from build123d import *

# Parameters (mm, degrees)
SKETCH_1_W                = 28
SKETCH_1_H                = 20
SKETCH_2_W                = 40
SKETCH_2_H                = 20
SKETCH_3_W                = 40
SKETCH_3_H                = 20
EXTRUDE_1_DEPTH           = 24
SKETCH_4_W                = 19
SKETCH_4_H                = 20
CUT_EXTRUDE_1_DEPTH       = 30
HOLE_WIZARD_M31_D         = 2.5
HOLE_WIZARD_M31_DEPTH     = 9
HOLE_WIZARD_M31_TIP       = 0.751075774
SKETCH_11_R               = 7
CUT_EXTRUDE_3_DEPTH       = 32
SKETCH_12_R               = 2
CUT_EXTRUDE_4_DEPTH       = 30
SKETCH_13_R               = 1.25
CUT_EXTRUDE_5_DEPTH       = 22
CUT_EXTRUDE_6_REACH       = 42
SKETCH_14_R               = 1.6
SKETCH_15_R               = 4
CUT_EXTRUDE_7_DEPTH       = 21
CHAMFER_1_SIZE            = 0.5
HOLE_WIZARD_M41_D         = 3.3
HOLE_WIZARD_M41_DEPTH     = 10
HOLE_WIZARD_M41_TIP       = 0.991420021
SKETCH_21_R               = 2.5
CUT_EXTRUDE_8_DEPTH       = 20
CUT_EXTRUDE_9_REACH       = 64
SKETCH_22_R               = 1.25
SKETCH_23_W               = 12.954085538
SKETCH_23_H               = 2
CUT_EXTRUDE_10_DEPTH      = 2
CUT_EXTRUDE_10_DEPTH_BACK = 2


with BuildPart() as part:
    # Эскиз1 → По сечениям1 section 0
    with BuildSketch(Plane(origin=(0, 0, 0), x_dir=(1, 0, 0), z_dir=(0, 1, 0))):
        with Locations((14, 10)):
            Rectangle(SKETCH_1_W, SKETCH_1_H)
    # Эскиз2 → По сечениям1 section 1
    with BuildSketch(Plane(origin=(0, -38, 0), x_dir=(1, 0, 0), z_dir=(0, 1, 0))):
        with Locations((20, 10)):
            Rectangle(SKETCH_2_W, SKETCH_2_H)
    loft()

    # Эскиз3 → Бобышка-Вытянуть1 (add)
    with BuildSketch(Plane.XZ.offset(38)):
        with Locations((20, -10)):
            Rectangle(SKETCH_3_W, SKETCH_3_H)
    extrude(amount=EXTRUDE_1_DEPTH)

    # Эскиз4 → Вырез-Вытянуть1 (cut)
    with BuildSketch(Plane.XZ.offset(62)):
        with Locations((9.5, -10)):
            Rectangle(SKETCH_4_W, SKETCH_4_H)
    extrude(amount=-CUT_EXTRUDE_1_DEPTH, mode=Mode.SUBTRACT)

    # Отверстие обработанное метчиком M31
    with Locations(Plane(origin=(0, 0, 0), x_dir=(1, 0, 0), z_dir=(0, 1, 0))):
        with Locations((3, 3), (3, 17), (24, 17), (24, 3)):
            Hole(HOLE_WIZARD_M31_D / 2, depth=HOLE_WIZARD_M31_DEPTH)
            with Locations((0, 0, -(HOLE_WIZARD_M31_DEPTH + HOLE_WIZARD_M31_TIP / 2))):  # 118° drill point
                Cone(0, HOLE_WIZARD_M31_D / 2, HOLE_WIZARD_M31_TIP, mode=Mode.SUBTRACT)

    # Эскиз11 → Вырез-Вытянуть3 (cut)
    with BuildSketch(Plane(origin=(0, 0, 0), x_dir=(1, 0, 0), z_dir=(0, 1, 0))):
        with Locations((10, 10)):
            Circle(SKETCH_11_R)
    extrude(amount=-CUT_EXTRUDE_3_DEPTH, mode=Mode.SUBTRACT)

    # Эскиз12 → Вырез-Вытянуть4 (cut)
    with BuildSketch(Plane(origin=(0, 0, 0), x_dir=(1, 0, 0), z_dir=(0, 1, 0))):
        with Locations((24, 10)):
            Circle(SKETCH_12_R)
    extrude(amount=-CUT_EXTRUDE_4_DEPTH, mode=Mode.SUBTRACT)

    # Эскиз13 → Вырез-Вытянуть5 (cut)
    with BuildSketch(Plane(origin=(0, -30, 0), x_dir=(1, 0, 0), z_dir=(0, 1, 0))):
        with Locations((24, 10)):
            Circle(SKETCH_13_R)
    extrude(amount=-CUT_EXTRUDE_5_DEPTH, mode=Mode.SUBTRACT)

    # Эскиз14 → Вырез-Вытянуть6 (cut, up to next)
    with BuildSketch(Plane.ZY, mode=Mode.PRIVATE) as cut_extrude_6_sk1:
        with Locations((-13, -17)):
            Circle(SKETCH_14_R)
    cut_extrude_6_tool1 = extrude(cut_extrude_6_sk1.sketch, amount=-CUT_EXTRUDE_6_REACH, mode=Mode.PRIVATE) & part.part
    add(cut_extrude_6_tool1.solids().sort_by_distance((0, -17, -13))[0], mode=Mode.SUBTRACT)
    # Эскиз14 → Вырез-Вытянуть6 (cut, up to next)
    with BuildSketch(Plane.ZY, mode=Mode.PRIVATE) as cut_extrude_6_sk2:
        with Locations((-7, -17)):
            Circle(SKETCH_14_R)
    cut_extrude_6_tool2 = extrude(cut_extrude_6_sk2.sketch, amount=-CUT_EXTRUDE_6_REACH, mode=Mode.PRIVATE) & part.part
    add(cut_extrude_6_tool2.solids().sort_by_distance((0, -17, -7))[0], mode=Mode.SUBTRACT)

    # Эскиз15 → Вырез-Вытянуть7 (cut)
    with BuildSketch(Plane(origin=(40, 0, 0), x_dir=(0, 0, -1), z_dir=(1, 0, 0))):
        with Locations((10, -52)):
            Circle(SKETCH_15_R)
    extrude(amount=-CUT_EXTRUDE_7_DEPTH, mode=Mode.SUBTRACT)

    # Фаска1
    chamfer_1_edges = [part.edges().sort_by_distance(p)[0] for p in [
        (40, -52, -6),
    ]]
    chamfer(chamfer_1_edges, length=CHAMFER_1_SIZE)

    # Отверстие обработанное метчиком M41
    with Locations(Plane(origin=(0, -62, 0), x_dir=(-1, 0, 0), z_dir=(0, -1, 0))):
        with Locations((-32, 10), (-24, 10)):
            Hole(HOLE_WIZARD_M41_D / 2, depth=HOLE_WIZARD_M41_DEPTH)
            with Locations((0, 0, -(HOLE_WIZARD_M41_DEPTH + HOLE_WIZARD_M41_TIP / 2))):  # 118° drill point
                Cone(0, HOLE_WIZARD_M41_D / 2, HOLE_WIZARD_M41_TIP, mode=Mode.SUBTRACT)

    # Эскиз21 → Вырез-Вытянуть8 (cut)
    with BuildSketch(Plane.XY):
        with Locations((32, -42)):
            Circle(SKETCH_21_R)
    extrude(amount=-CUT_EXTRUDE_8_DEPTH, mode=Mode.SUBTRACT)

    # Эскиз22 → Вырез-Вытянуть9 (cut, up to next)
    with BuildSketch(Plane.XZ.offset(62), mode=Mode.PRIVATE) as cut_extrude_9_sk1:
        with Locations((32, -10)):
            Circle(SKETCH_22_R)
    cut_extrude_9_tool1 = extrude(cut_extrude_9_sk1.sketch, amount=-CUT_EXTRUDE_9_REACH, mode=Mode.PRIVATE) & part.part
    add(cut_extrude_9_tool1.solids().sort_by_distance((32, -62, -10))[0], mode=Mode.SUBTRACT)

    # Эскиз23 → Вырез-Вытянуть10 (cut, two sides)
    with BuildSketch(Plane.XY.offset(-10)) as cut_extrude_10_sk:
        with Locations((17.522957231, -1)):
            Rectangle(SKETCH_23_W, SKETCH_23_H)
    extrude(amount=CUT_EXTRUDE_10_DEPTH, mode=Mode.SUBTRACT)
    extrude(cut_extrude_10_sk.sketch, amount=-CUT_EXTRUDE_10_DEPTH_BACK, mode=Mode.SUBTRACT)


solid = part.part
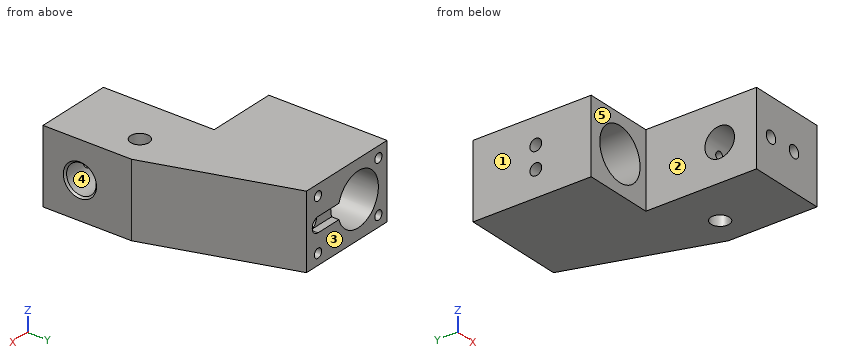
Can you work these out from the model? Positions are in its coordinate system, mm. Face numbers are marked on the shaded views. A direction names the side the tool comes from. Round coordinates to 2 decimals unless told otherwise and drop trailing zeros. Write each loop counter-clockwise with the first axis right and the second up, starting at its lowest first coordinate (ties: lowest second). Pieces come first, ordered by that corner, then holes. Notation, with made-up numbers: (-7.75, 67.5) - (-0.75, 67.5) arc R16 cw to (-0.75, 93.5) - close; hole circle Ø6 at (49.25, 16). An arc over 180 degrees is marked (long way). Write each question's results on one line, items separated by ' | '. Start each with the question number.
1) Suppose I cut it at A-A (y = -42). List the corners of the cut face in (x, z) for me.
2) Suppose I cut it at B-B (x = 10). List the corners of the cut face in (y, z) for me, and give its area (3 significant figures).
3) Please list where these lines run through material, in increasing order: line 1 (Y direction, x = 1.2, z = -13); line 2 (Z direction, x = 24, y = -7); line 3 (X direction, y = -45.35, z = -10).
4) Which directions (+Z, -Z, +X, -X, +Y, -Y) give clear straight access to the entire face, cutting with the end or side of a thin tool? Please do the marked faces 1 and 2.
5) For pin 1 Ø3.5 at (y, z) = (-17, -7) entering from +X; pin 2 Ø3 at (x, z) = (24, -10) entering from -Y; pin 3 Ø1 at (x, z) = (17, -9) entering from +Y; pin 4 Ø11 at (x, z) = (10, -10) entering from +Y, each with a flat end and sliding along its axis, tell me the tip position at first contact or that it passes through.
6) We'd pull the mould along Y, two halves only. Please class the marked faces 3, 4 and 5: released by +Y, released by -Y, zero draft, split by the parting line, or undercut.
7) Suppose I cut it at D-D (x = 32). List the corners of the cut face in (y, z) for me, and give its area (3 significant figures).
8) Suppose I cut it at C-C (x = 20). List the corners of the cut face in (y, z) for me.
Here are the results:
1) outline: (19, -20) - (29.5, -20) - (29.5, 0) - (19, 0) - close; (34.5, -20) - (40, -20) - (40, 0) - (34.5, 0) - close; hole circle Ø2.5 at (24, -10)
2) outline: (-32, -20) - (0, -20) - (0, -17) - (-32, -17) - close; (-32, -3) - (0, -3) - (0, 0) - (-32, 0) - close | area: 192 mm2
3) line 1: y = -32 to -18.6, -15.4 to 0 | line 2: z = -20 to -18.25, -15.75 to -12, -8 to -4.25, -1.75 to 0 | line 3: x = 19 to 22.75, 25.25 to 30.75, 33.25 to 40
4) face 1: +Z, -Z, -X, +Y, -Y | face 2: +Z, -Z, -X, -Y
5) pin 1: stops at x = 33.92 | pin 2: stops at y = -48.29 | pin 3: stops at y = -2 | pin 4: passes through
6) face 3: released by +Y | face 4: undercut | face 5: released by -Y
7) outline: (-62, -20) - (-44.5, -20) - (-44.5, -11.25) - (-48.2, -11.25) arc R4 cw to (-55.64, -11.65) - (-62, -11.65) - close; (-62, -8.35) - (-55.64, -8.35) arc R4 cw to (-48.2, -8.75) - (-44.5, -8.75) - (-44.5, 0) - (-62, 0) - close; (-39.5, -20) - (-12.67, -20) - (-12.67, 0) - (-39.5, 0) - close | area: 807 mm2
8) outline: (-62, -20) - (0, -20) - (0, -12) - (-2, -12) - (-2, -8) - (0, -8) - (0, 0) - (-62, 0) - close; hole circle Ø8 at (-52, -10)
